```python
from build123d import *

# Parameters (mm, degrees)
F0_W     = 6
F0_H     = 7
F0_R     = 1.6
F1_DEPTH = 4
F2_DEPTH = 2


# Not quite as in the source:
# - a feature names something its author has since deleted; it is built from what else it names


with BuildPart() as f1:
    # F0 (on Top) → F1 (new body)
    with BuildSketch(Plane.XY):
        Rectangle(F0_W, F0_H)
        Circle(F0_R, mode=Mode.SUBTRACT)
    extrude(amount=-F1_DEPTH)

    # F0 (on Top) → F2 (cut)
    with BuildSketch(Plane.XY):
        Rectangle(F0_W, F0_H)
        Circle(F0_R, mode=Mode.SUBTRACT)
    extrude(amount=-F2_DEPTH, mode=Mode.SUBTRACT)


solid = f1.part
```
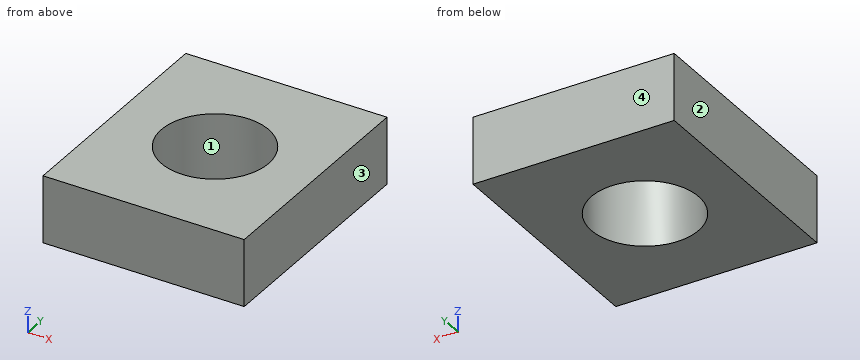
Source: CAD feature listing. Evaluate the final solid. Frame: model axes, mm. Face numbers are marked on the shaded views. Round coordinates to 2 decimals unless told otherwise and drop trailing zeros. Loops run counter-clockwise (first coordinate to the right, second up) from the corner with the lowest first, then second, coordinate; pieces in that order, holes last. Notation, with made-up numbers: M 31,-4 L 71,-4 A30 ccw 71,26 Z; hole C 17.5,55 d11. An arc over 180 degrees is marked long. Use a Markdown table: item, result. Add a question column.
1. Cut plane C-C, the plane z = -3.1. Output: boundary loops of the cut face in (x, y).
2. Cut plane A-A, the plane y = 0. Output: boundary loops of the cut face in (x, z).
3. Pull-direction query (X, two-part tool) for the marked faces 1, 2, 3 and 4; classes: +X half, -X half, draft (parallel to the pull), parting line (faces both ways), or undercut.
4. Ray query, line 1 along Y through (x, z) = (0, -2.5); line 2 along Y through (x, z) = (1, -2.15); line 3 along X through (y, z) = (0.5, -2.2). Return the intervals inside material, ascending. Write a range as [from, to].
5. Cut plane B-B, the plane x = 0. Output: boundary loops of the cut face in (y, z).
Solution:
| question | item | result |
|---|---|---|
| 1 | outline | M -3,-3.5 L 3,-3.5 L 3,3.5 L -3,3.5 Z; hole C 0,0 d3.2 |
| 2 | outline | M -3,-4 L -1.6,-4 L -1.6,-2 L -3,-2 Z; M 1.6,-4 L 3,-4 L 3,-2 L 1.6,-2 Z |
| 3 | face 1 | undercut |
| 3 | face 2 | -X half |
| 3 | face 3 | +X half |
| 3 | face 4 | draft |
| 4 | line 1 | y = [-3.5, -1.6], [1.6, 3.5] |
| 4 | line 2 | y = [-3.5, -1.25], [1.25, 3.5] |
| 4 | line 3 | x = [-3, -1.52], [1.52, 3] |
| 5 | outline | M -3.5,-4 L -1.6,-4 L -1.6,-2 L -3.5,-2 Z; M 1.6,-4 L 3.5,-4 L 3.5,-2 L 1.6,-2 Z |
